Design review of the part built by this model. Coordinates are the model's own, in mm. Face numbers are marked on the shaded views. A direction names the side the tool comes from. Round coordinates to 2 decimals unless told otherwise and drop trailing zeros. Order: outer loops, then holes, each group sorted by start corner. A loop starts at its lowest first (then second) coordinate and runs counter-clockwise, first axis right, second up. Notation, with made-up numbers: (0.5, 72.25) - (27.5, 72.25) arc R28 cw to (27.5, 105.25) - close; hole circle Ø3 at (-20.5, 27). An arc over 180 degrees is marked (long way). Write item = value, one per line.
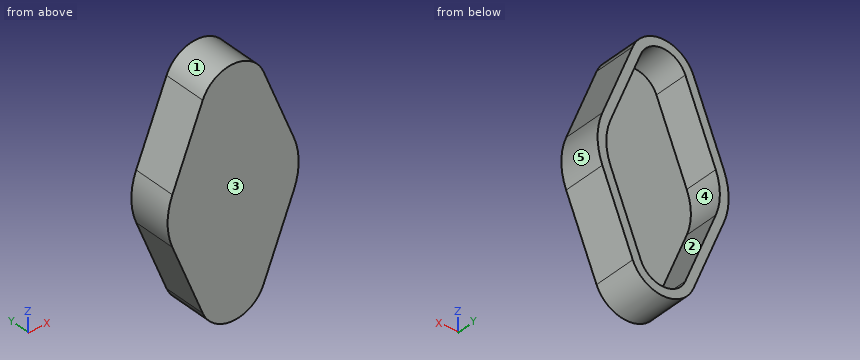
Autodesk Inventor part; units mm, degrees
ref_plane "YZ Plane" through (0, 0, 0) normal (1, 0, 0) x (0, 1, 0)
ref_plane "XZ Plane" through (0, 0, 0) normal (0, 1, 0) x (-1, 0, 0)
ref_plane "XY Plane" through (0, 0, 0) normal (0, 0, 1) x (1, 0, 0)
sketch "Sketch3" plane through (0, 0, 0) normal (0, 1, 0) x (-1, 0, 0)
  circle A0 centre (0, 0) radius 38.1
  circle A1 centre (0, -50.8) radius 19.05
  circle A2 centre (0, 50.8) radius 19.05
  line L0 (17.6598, 57.9438) -> (35.3196, 14.2875)
  line L1 (35.3196, -14.2875) -> (17.6598, -57.9438)
  line L2 (-17.6598, -57.9438) -> (-35.3196, -14.2875)
  line L3 (-17.6598, 57.9437) -> (-35.3196, 14.2875)
  dimension "d22" = 76.2
  dimension "d23" = 38.1
  dimension "d24" = 38.1
  dimension "d25" = 50.8
  dimension "d26" = 50.8
extrude "Extrusion2" add sketch "Sketch3" along normal blind 25.4
shell "Shell3" thickness 5.08 removed faces 1 at (-5.8866, 25.4, -28.8396)
properties part number "Diamond-Box"
Item 1: Insertion check: P1, Ø6, axis at x = 12, z = 4.5, coming from the +Y side; P2, Ø12, axis at x = -14.5, y = 22, coming from the +Z side; P3, Ø12, axis at y = 9, z = 34, coming from the +X side. Each pin has a flat end and moves straight along its axis. Give the tip position at first contact, or say it passes through.
Data:
P1 = 5.08
P2 = 67.85
P3 = 29.77
Item 2: For line 1 along Y through (x, z) = (-13.5, -41); line 2 along Z through (x, y) = (-11, 10); line 3 along X through (y, z) = (10.25, 13), list the stretches that pass through material, from the lowest coordinate up. Write a range as [from, to].
Data:
line_1 = [0, 5.08]
line_2 = [-66.35, -59.41], [59.41, 66.35]
line_3 = [-35.81, -30.36], [30.36, 35.81]
Item 3: Take a section at C-C, the plane y = 10. State the section outline as (x, z) points, and give its area (3 significant figures).
Data:
outline = (-35.32, -14.29) - (-17.66, -57.94) arc R19.05 ccw to (17.66, -57.94) - (35.32, -14.29) arc R38.1 ccw to (35.32, 14.29) - (17.66, 57.94) arc R19.05 ccw to (-17.66, 57.94) - (-35.32, 14.29) arc R38.1 ccw to start; hole (-30.61, -12.38) - (-12.95, -56.04) arc R13.97 ccw to (12.95, -56.04) - (30.61, -12.38) arc R33.02 ccw to (30.61, 12.38) - (12.95, 56.04) arc R13.97 ccw to (-12.95, 56.04) - (-30.61, 12.38) arc R33.02 ccw to start
area = 1,630 mm2
Item 4: Take a section at A-A, the plane z = 44. State the section outline as (x, y) points.
Data:
outline = (-23.3, 0) - (23.3, 0) - (23.3, 25.4) - (17.82, 25.4) - (17.82, 5.08) - (-17.82, 5.08) - (-17.82, 25.4) - (-23.3, 25.4) - close
Item 5: For the marked faces 1 and 2, list the 3-axis set-ups (+Z, -Z, +X, -X, +Y, -Y) from which the entire face can be reached by the end or side of a thin tool; tool diameter is ignored.
Data:
face_1 = +Z, +Y, -Y
face_2 = +Y
Item 6: The part is to be moulded in two halves that separate along X. For the marked faces 3, 4 and 5, say which applies: +X half, -X half, draft (parallel to the pull), parting line (faces both ways), or undercut.
Data:
face_3 = draft
face_4 = undercut
face_5 = +X half
Item 7: Take a section at B-B, the plane x = 21. State the section outline as (y, z) points, and give its area (3 significant figures).
Data:
outline = (0, -49.69) - (25.4, -49.69) - (25.4, -36.14) - (5.08, -36.14) - (5.08, 36.14) - (25.4, 36.14) - (25.4, 49.69) - (0, 49.69) - close
area = 1,060 mm2
